```python
from build123d import *

# Parameters (mm, degrees)
BOSS_EXTRUDE1_DEPTH      = 1
BOSS_EXTRUDE1_DEPTH_BACK = 2.5
BOSS_EXTRUDE2_DEPTH      = 2.5
BOSS_EXTRUDE3_DEPTH      = 1
BOSS_EXTRUDE4_DEPTH      = 1
CUT_EXTRUDE1_DEPTH       = 13.71154331


with BuildPart() as part:
    # Sketch1 → Boss-Extrude1 (new, two sides: drawn at the far end of the back side and taken through both)
    with BuildSketch(Plane.XY.offset(-BOSS_EXTRUDE1_DEPTH_BACK)):
        Polygon((8.082903769, 0), (4.041451884, 7), (-4.041451884, 7), (-8.082903769, 0), (-4.041451884, -7), (4.041451884, -7), align=None)
        Polygon((5.888972746, 0), (2.944486373, 5.1), (-2.944486373, 5.1), (-5.888972746, 0), (-2.944486373, -5.1), (2.944486373, -5.1), align=None, mode=Mode.SUBTRACT)
    extrude(amount=BOSS_EXTRUDE1_DEPTH + BOSS_EXTRUDE1_DEPTH_BACK)

    # Sketch3 → Boss-Extrude2 (add)
    with BuildSketch(Plane.XY):
        Polygon((5.888972746, 0), (2.944486373, 5.1), (-2.944486373, 5.1), (-5.888972746, 0), (-2.944486373, -5.1), (2.944486373, -5.1), align=None)
        Polygon((5.542562584, 0), (2.771281292, 4.8), (-2.771281292, 4.8), (-5.542562584, 0), (-2.771281292, -4.8), (2.771281292, -4.8), align=None, mode=Mode.SUBTRACT)
    extrude(amount=-BOSS_EXTRUDE2_DEPTH)

    # Sketch4 → Boss-Extrude3 (add)
    with BuildSketch(Plane(origin=(0, 0, -2.5), x_dir=(-1, 0, 0), z_dir=(0, 0, -1))):
        Polygon((9.237604307, 0), (4.618802154, 8), (-4.618802154, 8), (-9.237604307, 0), (-4.618802154, -8), (4.618802154, -8), align=None)
    extrude(amount=BOSS_EXTRUDE3_DEPTH)

    # Sketch5 → Boss-Extrude4 (add)
    with BuildSketch(Plane.XY.offset(-2.5)):
        Polygon((-4.618802154, 8), (-9.237604307, 0), (-4.618802154, -8), (4.618802154, -8), (9.237604307, 0), (4.618802154, 8), align=None)
        Polygon((-4.070319398, 7.05), (-8.140638796, 0), (-4.070319398, -7.05), (4.070319398, -7.05), (8.140638796, 0), (4.070319398, 7.05), align=None, mode=Mode.SUBTRACT)
    extrude(amount=BOSS_EXTRUDE4_DEPTH)

    # Sketch5<2> → Cut-Extrude1 (cut, through all)
    with BuildSketch(Plane.XY.offset(-2.5)):
        Polygon((4.041451884, -7), (8.082903769, 0), (4.041451884, 7), (-4.041451884, 7), (-8.082903769, 0), (-4.041451884, -7), align=None)
        Polygon((5.542562584, 0), (2.771281292, -4.8), (-2.771281292, -4.8), (-5.542562584, 0), (-2.771281292, 4.8), (2.771281292, 4.8), align=None, mode=Mode.SUBTRACT)
    extrude(amount=CUT_EXTRUDE1_DEPTH, mode=Mode.SUBTRACT)


solid = part.part
```
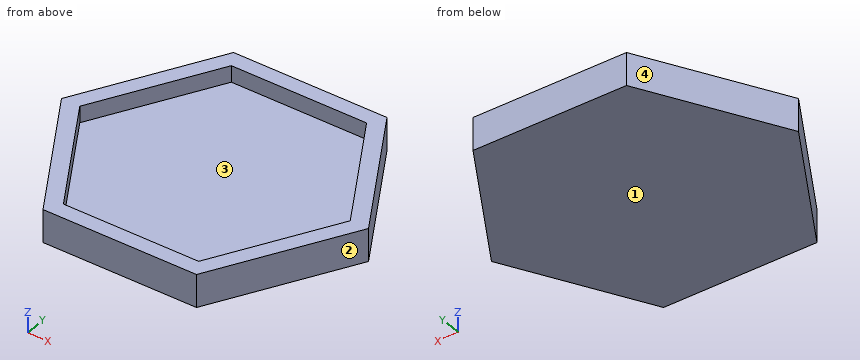
The listing builds one solid part. Answer for the finished solid, in the listing's coordinates (mm). Face numbers are marked on the shaded views. Round coordinates to 2 decimals unless told otherwise and drop trailing zeros. Order: outer loops, then holes, each group sorted by start corner. A loop starts at its lowest first (then second) coordinate and runs counter-clockwise, first axis right, second up. Notation, with made-up numbers: (43.5, 61) - (54.5, 61) arc R14 ccw to (54.5, 81) - close; hole circle Ø3 at (76, -30). An arc over 180 degrees is marked (long way). Put each result on its own line as item: value. Start each with the question number.
(1) Straight lines are drawn through the part: probe 1 along Y at (x, z) = (2, -1.85); probe 2 along Z at (x, y) = (-7, -0.25); probe 3 along X at (y, z) = (-7, -2.4). For each, find the intervals that lie inside material, in ascending order. Write a range as from..to.
(2) Find section C-C (y = 5.5). Give the vertices of the cut face in (x, z), plus the area to 3 significant figures.
(3) Find section A-A (z = -1.85). Give the vertices of the cut face in (x, y).
(4) Find section D-D (z = -3). Give the vertices of the cut face in (x, y).
(5) Determine the mould class of the marked faces 1, 2, 3 and 4 for opening direction Y: released by +Y, released by -Y, zero draft, split by the parting line, or undercut.
(6) Find section B-B (x = -2). Give the vertices of the cut face in (y, z).
(7) Given P1, Ø4, axis at x = 0, y = 3.5, coming from the +Z side; P2, Ø6, axis at x = 4.5, y = -4.5, coming from the +Z side, each flat-ended and moving along its own axis, determine where each tip first touches the part or whether it passes through.
Reply:
1. probe 1: -8..-7.05, 7.05..8
1. probe 2: -3.5..-2.5
1. probe 3: -5.2..-4.1, 4.1..5.2
2. outline: (-6.06, -3.5) - (6.06, -3.5) - (6.06, -1.5) - (4.97, -1.5) - (4.97, -2.5) - (-4.97, -2.5) - (-4.97, -1.5) - (-6.06, -1.5) - close
2. area: 14.3 mm^2
3. outline: (-9.24, 0) - (-4.62, -8) - (4.62, -8) - (9.24, 0) - (4.62, 8) - (-4.62, 8) - close; hole (-8.14, 0) - (-4.07, -7.05) - (4.07, -7.05) - (8.14, 0) - (4.07, 7.05) - (-4.07, 7.05) - close
4. outline: (-9.24, 0) - (-4.62, -8) - (4.62, -8) - (9.24, 0) - (4.62, 8) - (-4.62, 8) - close
5. face 1: zero draft
5. face 2: released by -Y
5. face 3: undercut
5. face 4: released by +Y
6. outline: (-8, -3.5) - (8, -3.5) - (8, -1.5) - (7.05, -1.5) - (7.05, -2.5) - (-7.05, -2.5) - (-7.05, -1.5) - (-8, -1.5) - close
7. P1: z = -2.5
7. P2: z = -1.5
